Autodesk Inventor part; units mm, degrees
ref_plane "YZ Plane" through (0, 0, 0) normal (1, 0, 0) x (0, 1, 0)
ref_plane "XZ Plane" through (0, 0, 0) normal (0, 1, 0) x (-1, 0, 0)
ref_plane "XY Plane" through (0, 0, 0) normal (0, 0, 1) x (1, 0, 0)
sketch "Sketch1" plane through (0, 0, 0) normal (0, 1, 0) x (-1, 0, 0)
  line L0 (0, 0) -> (69, 0)
  line L1 (69, 0) -> (69, -92)
  line L2 (69, -92) -> (0, -92)
  line L3 (0, -92) -> (0, 0)
  dimension "d0" = 69
  dimension "d1" = 92
extrude "Extrusion1" add sketch "Sketch1" along normal blind 1
sketch "Sketch2" plane through (0, 1, 0) normal (0, 1, 0) x (1, 0, 0)
  line L0 (-69, 0) -> (0, 0)
  line L1 (0, 0) -> (0, 92)
  line L2 (0, 92) -> (-69, 92)
  line L3 (-69, 92) -> (-69, 0)
  line L4 (-68, 1) -> (-1, 1)
  line L5 (-1, 1) -> (-1, 91)
  line L6 (-1, 91) -> (-68, 91)
  line L7 (-68, 91) -> (-68, 1)
  line L8 (-67.5, 1) -> (-67.5, 91)
  line L9 (-1.5, 1) -> (-1.5, 91)
  dimension "d4" = 1
  dimension "d5" = 0.5
  dimension "d6" = 0.5
extrude "Extrusion2" add sketch "Sketch2" along normal blind 5 contours L3 L2 L1 L0 | L7 L6 L8 L4 | L9 L6 L5 L4
sketch "Sketch3" plane through (0, 1, 0) normal (0, 1, 0) x (1, 0, 0)
  line L0 (-67.5, 91) -> (-67.5, 1)
  line L1 (-67.5, 1) -> (-1.5, 1)
  line L2 (-1.5, 1) -> (-1.5, 91)
  line L3 (-1.5, 91) -> (-67.5, 91)
  line L4 (-67.5, 1) -> (-1.5, 1)
  line L5 (-66.5, 1) -> (-66.5, 91)
  line L6 (-2.5, 1) -> (-2.5, 91)
  point P0 (0, 0)
  dimension "d9" = 1
  dimension "d10" = 1
extrude "Extrusion3" add sketch "Sketch3" along normal blind 12 contours L3 L5 L1 L0 | L3 L2 L1 L6
sketch "Sketch4" plane through (-1.5, 6, -91) normal (1, 0, 0) x (0, 0, -1)
  line L0 (-90, 0) -> (-90, 7)
  line L1 (-90, 4) -> (-90, 5)
  line L2 (0, 0) -> (0, 7)
  line L3 (-90, 7) -> (0, 7)
  line L4 (-60, 5) -> (-30, 5)
  line L5 (-30, 5) -> (-30, 4)
  line L6 (-30, 4) -> (-60, 4)
  line L7 (-60, 4) -> (-60, 5)
  line L8 (0, 0) -> (-90, 0)
  point P0 (-91, -6)
  dimension "d21" = 1
  dimension "d22" = 2
  dimension "d23" = 4
  dimension "d24" = 30
  dimension "d25" = 30
ref_plane "Work Plane1" through (-34.5, 0, 0) normal (1, 0, 0) x (0, 0, -1)
extrude "Extrusion5" add sketch "Sketch4" along normal blind 1 contours L4 L5 L6 L7
mirror "Mirror2" about plane through (-34.5, 0, 0) normal (1, 0, 0) of "Extrusion5"
sketch "Sketch5" plane through (0, 0, 0) normal (1, 0, 0) x (0, 0, -1)
  line L0 (92, 0) -> (0, 0)
  line L1 (92, 0) -> (92, 6)
  line L2 (0, 6) -> (92, 6)
  line L3 (0, 0) -> (0, 6)
extrude "Extrusion6" add sketch "Sketch5" along normal blind 1.5
sketch "Sketch6" plane through (-69, 0, -92) normal (-1, 0, 0) x (0, 0, 1)
  line L0 (92, 0) -> (0, 0)
  line L1 (92, 0) -> (92, 6)
  line L2 (0, 6) -> (92, 6)
  line L3 (0, 0) -> (0, 6)
extrude "Extrusion7" add sketch "Sketch6" along normal blind 1.5
properties part number "top2"
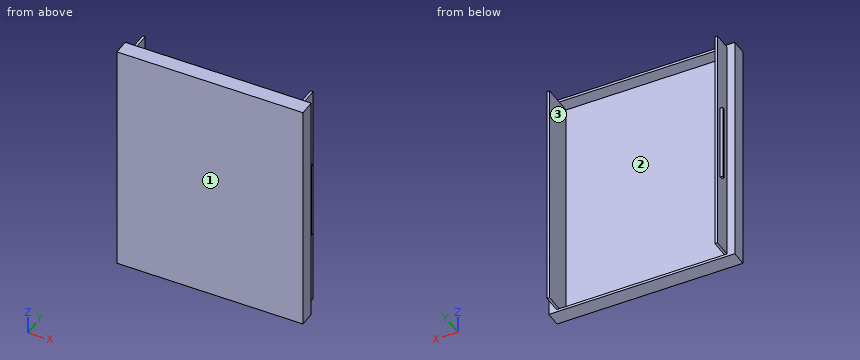
Could you check a few things on this model? Use its own coordinates, in mm. Face numbers are marked on the shaded views. Round coordinates to 2 decimals unless told otherwise and drop trailing zeros. Loops run counter-clockwise (first coordinate to the right, second up) from the corner with the lowest first, then second, coordinate; pieces in that order, holes last.
Q1. I want a section at B-B (x = -38). Write out the boundary of the cut face in (y, z), and give its area (3 significant figures).
Q2. For P1, Ø0.8, axis at x = -1, z = -41.5, coming from the +Y side; P2, Ø0.8, axis at x = -2, y = 10, coming from the +Z side; P3, Ø3, axis at y = 9, z = -47.5, coming from the +X side, each with a flat end and sliding along its axis, tell me the tip position at first contact or that it passes through.
Q3. I want a section at A-A (y = 7.5). Write out the boundary of the cut face in (x, z).
Q4. I want a section at C-C (z = -39.5). Write out the boundary of the cut face in (x, y).
Q5. Thinking about a two-plate mould opening in X: for the marked faces 1, 2 and 3, which applies, pulls with the +X half, pulls with the -X half, needs draft (parallel to the pull), parting line crosses it, or undercut?
Q6. I want a section at D-D (y = 2). Write out the boundary of the cut face in (x, z).
Q7. Please list where these lines run through material, in increasing order: L1, parallel to X at y = 8.75, z = -22; L2, parallel to X at y = 3.5, z = -11.5; L3, parallel to Y at x = -1, z = -59.
Answer below:
1. outline: (0, -92) - (6, -92) - (6, -91) - (1, -91) - (1, -1) - (6, -1) - (6, 0) - (0, 0) - close
1. area: 102 mm2
2. P1: stops at y = 11
2. P2: stops at z = -1
2. P3: stops at x = -0.5
3. outline: (-67.5, -91) - (-66.5, -91) - (-66.5, -1) - (-67.5, -1) - close; (-2.5, -91) - (-1.5, -91) - (-1.5, -1) - (-2.5, -1) - close
4. outline: (-70.5, 0) - (1.5, 0) - (1.5, 6) - (-1.5, 6) - (-1.5, 10) - (-0.5, 10) - (-0.5, 11) - (-1.5, 11) - (-1.5, 13) - (-2.5, 13) - (-2.5, 1) - (-66.5, 1) - (-66.5, 13) - (-67.5, 13) - (-67.5, 11) - (-68.5, 11) - (-68.5, 10) - (-67.5, 10) - (-67.5, 6) - (-70.5, 6) - close
5. face 1: needs draft
5. face 2: undercut
5. face 3: undercut
6. outline: (-70.5, -92) - (1.5, -92) - (1.5, 0) - (-70.5, 0) - close; hole (-66.5, -91) - (-2.5, -91) - (-2.5, -1) - (-66.5, -1) - close
7. L1: x = -67.5 to -66.5, -2.5 to -1.5
7. L2: x = -70.5 to -66.5, -2.5 to 1.5
7. L3: y = 0 to 6, 10 to 11
